Could you check a few things on this model? Use its own coordinates, in mm. A direction names the side the tool comes from. Round coordinates to 2 decimals unless told otherwise and drop trailing zeros. Loops run counter-clockwise (first coordinate to the right, second up) from the corner with the lowest first, then second, coordinate; pieces in that order, holes last.
from build123d import *

# Parameters (mm, degrees)
SKETCH2_W           = 33
SKETCH2_H           = 17.000000000000007
BOSS_EXTRUDE1_DEPTH = 2
FILLET1_R           = 8
FILLET2_R           = 8
CHAMFER1_SIZE       = 2
CUT_EXTRUDE2_DEPTH  = 12
SKETCH6_W           = 1.2612446076729746
SKETCH6_H           = 17.000000000000007
BOSS_EXTRUDE3_DEPTH = 2
SKETCH8_W           = 37.024907352098374
SKETCH8_H           = 22.564000776868035
BOSS_EXTRUDE4_DEPTH = 1.3
FILLET4_R           = 2
FILLET5_R           = 2
FILLET6_R           = 2
FILLET7_R           = 2
CHAMFER2_SIZE       = 2
CHAMFER3_SIZE       = 2
CHAMFER4_SIZE       = 2
CHAMFER5_SIZE       = 2


with BuildPart() as part:
    # Sketch2 → Boss-Extrude1 (new body)
    with BuildSketch(Plane(origin=(0, 0, 0), x_dir=(1, 0, 0), z_dir=(0, 1, 0))):
        Polygon((-15.000000000000073, 76.00000000000003), (15.000000000000004, 76.00000000000003), (57.894125564998674, 58.48538895430336), (57.894125564998674, 27.05184462316343), (52.49999999999998, 18.118100444839456), (-52.50000000000002, 18.118100444839435), (-57.89412556499873, 27.051844623163408), (-57.894125564998745, 58.48538895430333), align=None)
        with Locations((11.999999999999982, 36.50000000000003)):
            Rectangle(SKETCH2_W, SKETCH2_H, mode=Mode.SUBTRACT)
    extrude(amount=BOSS_EXTRUDE1_DEPTH)

    # Fillet1
    fillet1_edges = [part.edges().sort_by_distance(p)[0] for p in [
        (57.894125564998674, 1, -58.48538895430336),
    ]]
    fillet(fillet1_edges, radius=FILLET1_R)

    # Fillet2
    fillet2_edges = [part.edges().sort_by_distance(p)[0] for p in [
        (-57.894125564998745, 1, -58.48538895430333),
    ]]
    fillet(fillet2_edges, radius=FILLET2_R)

    # Chamfer1
    chamfer1_edges = [part.edges().sort_by_distance(p)[0] for p in [
        (-2.132e-14, 2, -18.118100444839445),
    ]]
    chamfer(chamfer1_edges, length=CHAMFER1_SIZE - 0.0001)  # a hair under: the kernel refuses the full size

    # Sketch3 → Cut-Extrude2 (cut)
    with BuildSketch(Plane(origin=(0, 2, 0), x_dir=(1, 0, 0), z_dir=(0, 1, 0))):
        Polygon((-7.894125564998744, 48.60000000000001), (-7.894125564998744, 28.000000000000025), (-4.500000000000018, 28.000000000000025), (-4.500000000000018, 45.00000000000003), (-4.500000000000016, 48.60000000000002), align=None)
        Polygon((-4.500000000000018, 45.00000000000003), (27.238755392327008, 45.00000000000003), (27.238755392327008, 48.600000000000016), (-4.500000000000016, 48.60000000000002), align=None)
    extrude(amount=-CUT_EXTRUDE2_DEPTH, mode=Mode.SUBTRACT)

    # Sketch6 → Boss-Extrude3 (add)
    with BuildSketch(Plane(origin=(0, 2, 0), x_dir=(1, 0, 0), z_dir=(0, 1, 0))):
        with Locations((27.869377696163497, 36.50000000000003)):
            Rectangle(SKETCH6_W, SKETCH6_H)
    extrude(amount=-BOSS_EXTRUDE3_DEPTH)

    # Sketch8 → Boss-Extrude4 (add)
    with BuildSketch(Plane(origin=(0, 2, 0), x_dir=(1, 0, 0), z_dir=(0, 1, 0))):
        with Locations((9.826111603405227, 38.39621794248441)):
            Rectangle(SKETCH8_W, SKETCH8_H)
        Polygon((-7.894125564998744, 48.60000000000001), (27.238755392327008, 48.600000000000016), (27.238755392327008, 28.000000000000025), (-7.894125564998744, 28.000000000000025), align=None, mode=Mode.SUBTRACT)
    extrude(amount=BOSS_EXTRUDE4_DEPTH)

    # Fillet4
    fillet4_edges = [part.edges().sort_by_distance(p)[0] for p in [
        (-8.68634207264396, 2.65, -49.67821833091842),
    ]]
    fillet(fillet4_edges, radius=FILLET4_R)

    # Fillet5
    fillet5_edges = [part.edges().sort_by_distance(p)[0] for p in [
        (28.338565279454414, 2.65, -49.67821833091842),
    ]]
    fillet(fillet5_edges, radius=FILLET5_R)

    # Fillet6
    fillet6_edges = [part.edges().sort_by_distance(p)[0] for p in [
        (28.338565279454414, 2.65, -27.11421755405039),
    ]]
    fillet(fillet6_edges, radius=FILLET6_R)

    # Fillet7
    fillet7_edges = [part.edges().sort_by_distance(p)[0] for p in [
        (-8.68634207264396, 2.65, -27.11421755405039),
    ]]
    fillet(fillet7_edges, radius=FILLET7_R)

    # Chamfer2
    chamfer2_edges = [part.edges().sort_by_distance(p)[0] for p in [
        (27.238755392327008, 0, -38.30000000000002),
    ]]
    chamfer(chamfer2_edges, length=CHAMFER2_SIZE)

    # Chamfer3
    chamfer3_edges = [part.edges().sort_by_distance(p)[0] for p in [
        (10.672314913664133, 0, -28.000000000000025),
    ]]
    chamfer(chamfer3_edges, length=CHAMFER3_SIZE)

    # Chamfer4
    chamfer4_edges = [part.edges().sort_by_distance(p)[0] for p in [
        (-7.894125564998744, 0, -37.30000000000002),
    ]]
    chamfer(chamfer4_edges, length=CHAMFER4_SIZE)

    # Chamfer5
    chamfer5_edges = [part.edges().sort_by_distance(p)[0] for p in [
        (9.672314913664131, 0, -48.60000000000009),
    ]]
    chamfer(chamfer5_edges, length=CHAMFER5_SIZE)


solid = part.part
Item 1: We'd pull the mould along X, two halves only. Please class faces 6 (the flat face through (-8.88, 1.014, -38.472)), 7 (the flat face through (-57.894, 1, -40)), 8 (the flat face through (57.894, 1, -40)): released by +X, released by -X, zero draft, split by the parting line, or undercut.
Results list:
face 6: undercut
face 7: released by -X
face 8: released by +X
Item 2: If we section it at C-C, the plane z = -43: Please give me the cut outline in (x, y), then the cut area to 3 significant figures.
Results list:
outline: (-57.89, 0) - (-9.89, 0) - (-7.89, 2) - (-7.89, 3.3) - (-8.69, 3.3) - (-8.69, 2) - (-57.89, 2) - close; (27.24, 2) - (29.24, 0) - (57.89, 0) - (57.89, 2) - (28.34, 2) - (28.34, 3.3) - (27.24, 3.3) - close
area: 160 mm2
Item 3: If we section it at A-A, the plane y = 2.6: Please give me the cut outline in (x, z), then the cut area to 3 significant figures.
Results list:
outline: (-8.69, -47.68) arc R2 ccw to (-6.69, -49.68) - (26.34, -49.68) arc R2 ccw to (28.34, -47.68) - (28.34, -29.11) arc R2 ccw to (26.34, -27.11) - (-6.69, -27.11) arc R2 ccw to (-8.69, -29.11) - close; hole (-7.89, -48.6) - (27.24, -48.6) - (27.24, -28) - (-7.89, -28) - close
area: 108 mm2
Item 4: Will these pins go through, and if not, where does the flat tip stop? pin 1 (1.4 mm diameter, centred on y = 3, z = -40.5, fed in from -X); pin 2 (1 mm diameter, centred on x = -19.5, y = 1.5, fed in from -Z); pin 3 (1.4 mm diameter, centred on y = 2.5, z = -39.5, fed in from +X); pin 4 (1 mm diameter, centred on y = 1.5, z = -65, fed in from +X).
Results list:
pin 1: stops at x = -8.69
pin 2: stops at z = -74.37
pin 3: stops at x = 57.89
pin 4: stops at x = 43.16
Item 5: If I drill on line 1 along Z through (x, y) = (10, 2.45); line 2 along Y through (x, z) = (-36.5, -41); line 3 along Z through (x, y) = (23, 1.6), over which ranges is the centre line in solid material (lowest first)?
Results list:
line 1: z = -49.68 to -48.6, -28 to -27.11
line 2: y = 0 to 2
line 3: z = -72.73 to -49, -27.6 to -19.72
Item 6: For faces 1 (the cylindrical face through (27.737, 2.659, -49.108)), 2 (the cylindrical face through (-8.116, 2.659, -49.077)), 3 (the flat face through (9.7, 3.3, -27.6)), 4 (the cylindrical face through (28, 3, -28)), 5 (the cylindrical face through (-8.1, 2.7, -27.7)), which set-ups out of +Z, -Z, +X, -X, +Y, -Y let a thin tool reach every point of the face, with its end or its side?
Results list:
face 1: -Z, +X, +Y
face 2: -Z, -X, +Y
face 3: +Z, -Z, +X, -X, +Y
face 4: +Z, +X, +Y
face 5: +Z, -X, +Y
